Read the model definition and answer for the solid it produces. Units are mm, in the model's axes. Give positions to 0.01 mm unless a question says otherwise; leave off trailing zeros. Order: outer loops, then holes, each group sorted by start corner. A loop starts at its lowest first (then second) coordinate and runs counter-clockwise, first axis right, second up.
Item 1: A cutting plane is placed at A-A (x = 7.5). Write down the section's boundary in (y, z).
Item 2: A cutting plane is placed at C-C (y = -7). Write down the section's boundary in (x, z).
Item 3: A cutting plane is placed at B-B (z = 45). Write down the section's boundary in (x, y), plus the area to 3 significant figures.
Item 4: The mould has two halves that part along Z. Classify faces 1 (the face through (0, -12, 44)), 2 (the face through (12, -7, 5)), 3 (the face through (11.832, -6.479, 18.966)): +Z half, -Z half, draft (parallel to the pull), parting line (faces both ways), or undercut.
Item 5: Find the intervals of material crossed by line 1 along Z through (x, y) = (8.75, -7); line 2 along Z through (x, y) = (16.75, -4.25); line 3 along Y through (x, z) = (14.5, 78), in increasing order.
from build123d import *

# Parameters (mm, degrees)
SKETCH_1_W          = 24
SKETCH_1_H          = 14
EXTRUDE_1_DEPTH     = 90
SKETCH_2_R          = 4
CUT_EXTRUDE_1_DEPTH = 90
SKETCH_3_W          = 5
SKETCH_3_H          = 14
CUT_EXTRUDE_2_DEPTH = 95.191294715


with BuildPart() as part:
    # 草图1 → 拉伸1 (new body)
    with BuildSketch(Plane.XY):
        with Locations((12, -7)):
            Rectangle(SKETCH_1_W, SKETCH_1_H)
    extrude(amount=EXTRUDE_1_DEPTH)

    # 草图2 → 切除-拉伸1 (cut)
    with BuildSketch(Plane.ZY):
        with Locations(Location((15, -7, 0), (0, 0, 270))):
            Circle(SKETCH_2_R)
        with Locations(Location((45, -7, 0), (0, 0, 270))):
            Circle(SKETCH_2_R)
        with Locations(Location((75, -7, 0), (0, 0, 270))):
            Circle(SKETCH_2_R)
    extrude(amount=-CUT_EXTRUDE_1_DEPTH, mode=Mode.SUBTRACT)

    # 草图3 → 切除-拉伸2 (cut, through all)
    with BuildSketch(Plane(origin=(24, 0, 0), x_dir=(0, 0, -1), z_dir=(1, 0, 0))):
        with Locations((-87.5, -7)):
            Rectangle(SKETCH_3_W, SKETCH_3_H)
        with Locations((-2.5, -7)):
            Rectangle(SKETCH_3_W, SKETCH_3_H)
    extrude(amount=-CUT_EXTRUDE_2_DEPTH, mode=Mode.SUBTRACT)


solid = part.part
Response values:
1. outline: (-14, 5) - (0, 5) - (0, 85) - (-14, 85) - close; hole circle Ø8 at (-7, 15); hole circle Ø8 at (-7, 45); hole circle Ø8 at (-7, 75)
2. outline: (0, 5) - (24, 5) - (24, 11) - (0, 11) - close; (0, 19) - (24, 19) - (24, 41) - (0, 41) - close; (0, 49) - (24, 49) - (24, 71) - (0, 71) - close; (0, 79) - (24, 79) - (24, 85) - (0, 85) - close
3. outline: (0, -14) - (24, -14) - (24, -11) - (0, -11) - close; (0, -3) - (24, -3) - (24, 0) - (0, 0) - close
3. area: 144 mm2
4. face 1: draft
4. face 2: -Z half
4. face 3: undercut
5. line 1: z = 5 to 11, 19 to 41, 49 to 71, 79 to 85
5. line 2: z = 5 to 12.1, 17.9 to 42.1, 47.9 to 72.1, 77.9 to 85
5. line 3: y = -14 to -9.65, -4.35 to 0
